Job drawing, mm, ordinate dimensions from the low corner. One solid piece. A direction names the side the tool comes from. Give positions to 0.01 mm unless a question says otherwise; leave off trailing zeros. Order: outer loops, then holes, each group sorted by start corner. A loop starts at its lowest first (then second) coordinate and runs counter-clockwise, first axis right, second up. Notation, with made-up numbers: (22.5, 34.5) - (61.5, 34.5) arc R31 ccw to (61.5, 66.5) - close; hole circle Ø1 at (53.25, 28.25). An arc over 180 degrees is marked (long way). Use one line per item in the form item = value. Start each with the question number.
1. Tool access for the marked faces 1, 2, 3 and 4: list every direction of +Z, -Z, +X, -X, +Y, -Y with a clear straight run to the whole face (end or side of a thin tool).
2. Pin check, flat tips, straight feed: P1, Ø3, axis at x = 160.5, y = 113.5, coming from the +Z side; P2, Ø12, axis at y = 90, z = 124, coming from the -X side; P3, Ø12, axis at y = 91, z = 172, coming from the +X side. Stop position of each tip, or through.
3. Band-saw the part on A-A, the plane y = 100. List the corners of the cut face in (x, z).
4. Band-saw the part on D-D, the plane y = 134.5. List the corners of the cut face in (x, z).
5. Drill centre lines: line 1 (X direction, y = 100, z = 112); line 2 (Y direction, x = 84, z = 184). Where is each one in solid material? Low to high.
6. Band-saw the part on C-C, the plane z = 144.5. List the corners of the cut face in (x, y).
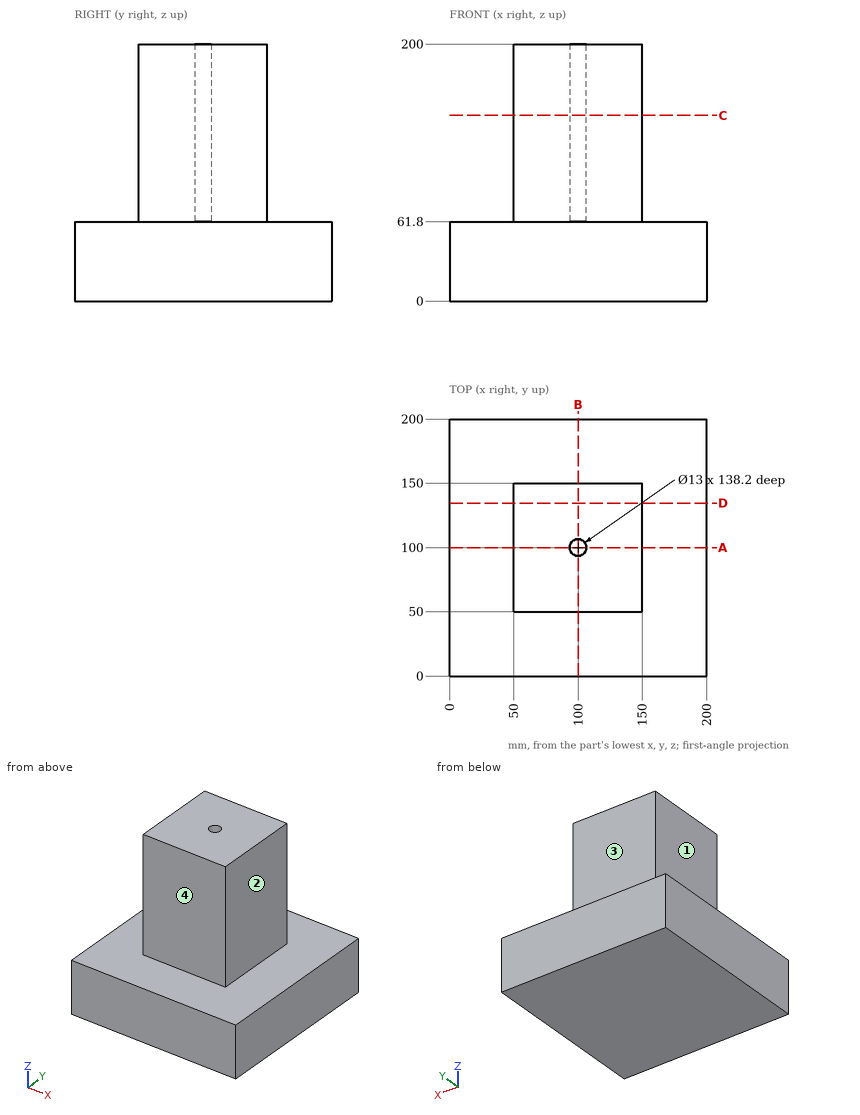
From the geometry:
q1.face_1 = +Z, -X, +Y, -Y
q1.face_2 = +Z, +X, +Y, -Y
q1.face_3 = +Z, +X, -X, +Y
q1.face_4 = +Z, +X, -X, -Y
q2.P1 = 61.8
q2.P2 = 50
q2.P3 = 150
q3.outline = (0, 0) - (200, 0) - (200, 61.8) - (150, 61.8) - (150, 200) - (106.5, 200) - (106.5, 61.8) - (93.5, 61.8) - (93.5, 200) - (50, 200) - (50, 61.8) - (0, 61.8) - close
q4.outline = (0, 0) - (200, 0) - (200, 61.8) - (150, 61.8) - (150, 200) - (50, 200) - (50, 61.8) - (0, 61.8) - close
q5.line_1 = 50 to 93.5, 106.5 to 150
q5.line_2 = 50 to 150
q6.outline = (50, 50) - (150, 50) - (150, 150) - (50, 150) - close; hole circle Ø13 at (100, 100)
